Read the model definition and answer for the solid it produces. Units are mm, in the model's axes. Give positions to 0.01 mm unless a question says otherwise; leave off trailing zeros. Write each loop counter-clockwise with the first axis right and the second up, starting at its lowest first coordinate (ties: lowest second). Pieces come first, ordered by that corner, then holes. Notation, with made-up numbers: M 6,52.5 L 33,52.5 A7 ccw 33,62.5 Z; hole C -28.5,2 d9. An arc over 180 degrees is marked long. Put each result on its own line as item: value.
from build123d import *

# Parameters (mm, degrees)
BOSS_EXTRUDE1_DEPTH = 3.175
SKETCH3_W           = 149.303507008
SKETCH3_H           = 288.678903575
CUT_EXTRUDE1_DEPTH  = 101.601825752
SKETCH4_W           = 3.302
SKETCH4_H           = 7.449124121
SKETCH4_H_2         = 9.965839279
CUT_EXTRUDE2_DEPTH  = 4.175


with BuildPart() as part:
    # Sketch2 → Boss-Extrude1 (new body)
    with BuildSketch(Plane.XY):
        with BuildLine():
            ThreePointArc((-1.783927604, 106.664181958), (-86.289926541, 57.796410124), (-89.548347912, -39.767444199))
            ThreePointArc((-89.548347912, -39.767444199), (-89.139366423, -40.557656379), (-88.723411943, -41.344220438))
            ThreePointArc((-88.723411943, -41.344220438), (-88.300763494, -42.126623343), (-87.87121564, -42.905259753))
            ThreePointArc((-87.87121564, -42.905259753), (0, -94.523651503), (87.87121564, -42.905259753))
            ThreePointArc((87.87121564, -42.905259753), (88.300763494, -42.126623343), (88.723411943, -41.344220438))
            ThreePointArc((88.723411943, -41.344220438), (89.139366423, -40.557656379), (89.548347912, -39.767444199))
            ThreePointArc((89.548347912, -39.767444199), (86.289926541, 57.796410124), (1.783927604, 106.664181958))
            ThreePointArc((1.783927604, 106.664181958), (0.891998866, 106.676045412), (0, 106.68))
            ThreePointArc((0, 106.68), (-0.891998866, 106.676045412), (-1.783927604, 106.664181958))
        make_face()
        with BuildLine():
            ThreePointArc((-7.652045127, 93.646303016), (0, -81.823651503), (7.652045127, 93.646303016))
            ThreePointArc((7.652045127, 93.646303016), (4.717664566, 93.853310885), (1.778000524, 93.962016248))
            ThreePointArc((1.778000524, 93.962016248), (0.889045735, 93.975503947), (0, 93.98))
            ThreePointArc((0, 93.98), (-0.889045735, 93.975503947), (-1.778000524, 93.962016248))
            ThreePointArc((-1.778000524, 93.962016248), (-4.717664566, 93.853310885), (-7.652045127, 93.646303016))
        make_face(mode=Mode.SUBTRACT)
    extrude(amount=-BOSS_EXTRUDE1_DEPTH)

    # Sketch3 → Cut-Extrude1 (cut, through all)
    with BuildSketch(Plane(origin=(0, 0, 0), x_dir=(0, 0, -1), z_dir=(1, 0, 0))):
        with Locations((2.160275602, 8.369276658)):
            Rectangle(SKETCH3_W, SKETCH3_H)
    extrude(amount=CUT_EXTRUDE1_DEPTH, mode=Mode.SUBTRACT)

    # Sketch4 → Cut-Extrude2 (cut, through all)
    with BuildSketch(Plane.XY):
        Polygon((-88.109110822, 62.776111712), (-78.996562371, 57.51497941), (-80.761862371, 54.45739012), (-89.874410822, 59.718522421), align=None)
        Polygon((-84.09504483, -36.64600391), (-82.32974483, -39.7035932), (-90.457535691, -44.396175442), (-92.222835691, -41.338586151), align=None)
        with Locations((-1.651, -91.898213564)):
            Rectangle(SKETCH4_W, SKETCH4_H)
        with Locations((-1.651, 105.31291964)):
            Rectangle(SKETCH4_W, SKETCH4_H_2)
    extrude(amount=-CUT_EXTRUDE2_DEPTH, mode=Mode.SUBTRACT)


solid = part.part
(1) Given pin 1 Ø1 at (y, z) = (-90, -1) entering from +X; pin 2 Ø1 at (x, z) = (-2.5, -2) entering from -Y, each flat-ended and moving along its own axis, determine where each tip first touches the part or whether it passes through.
Result:
pin 1: stops at x = -3.3
pin 2: stops at y = -88.17
(2) Section C-C on x = -54 is taken. Determine the outline of the cut face in (y, z) (1 decimal).
Result:
outline: M -78.8,-3.2 L -63.3,-3.2 L -63.3,0 L -78.8,0 Z; M 75.4,-3.2 L 91,-3.2 L 91,0 L 75.4,0 Z
(3) Section A-A on x = -29 is taken. Determine the outline of the cut face in (y, z) (3 decimals).
Result:
outline: M -90.253,-3.175 L -76.902,-3.175 L -76.902,0 L -90.253,0 Z; M 89.058,-3.175 L 102.41,-3.175 L 102.41,0 L 89.058,0 Z
(4) Section D-D on y = 69 is taken. Determine the outline of the cut face in (x, z) (3 decimals), and give its area (3 significant figures).
Result:
outline: M -78.496,-3.175 L -61.381,-3.175 L -61.381,0 L -78.496,0 Z
area: 54.3 mm²
(5) Straight lines are drawn through the part: line 1 along Y through (x, z) = (-6.5, -0.85); line 2 along Y through (x, z) = (-62, -1.6); line 3 along X through (y, z) = (37, -0.9). For each, find the intervals that lie inside material, in ascending order. Write a range as from..to.
Result:
line 1: y = -94.31..-81.58, 93.74..106.47
line 2: y = -73.15..-56.23, 68.39..85.3
line 3: x = -95.73..-82.28
